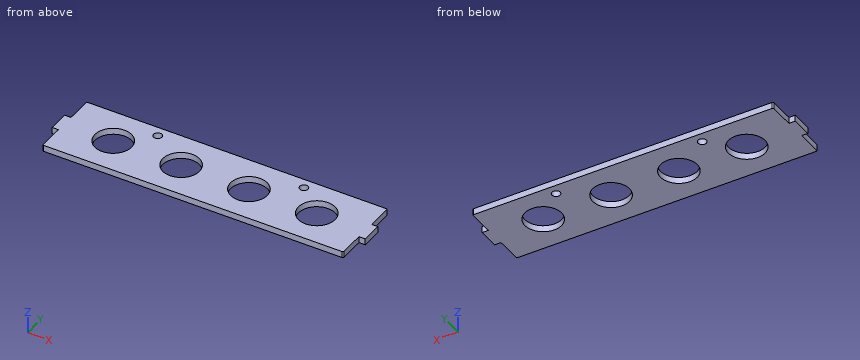
```python
from build123d import *

# Parameters (mm, degrees)
SKETCH1_W   = 300
SKETCH1_H   = 70
FRONT_DEPTH = 6
SKETCH2_W   = 6
SKETCH2_H   = 25
SKETCH2_R   = 4
MOUNT_DEPTH = 309.116860947
FILLET_2_R  = 1
SKETCH3_R   = 17.5
LITE_DEPTH  = 309.116860947


with BuildPart() as part:
    # Sketch1 → front (new body)
    with BuildSketch(Plane.XY):
        with Locations((150, 35)):
            Rectangle(SKETCH1_W, SKETCH1_H)
    extrude(amount=-FRONT_DEPTH)

    # Sketch2 → mount (cut, through all)
    with BuildSketch(Plane.XY):
        with Locations((3, 57.5)):
            Rectangle(SKETCH2_W, SKETCH2_H)
        with Locations((3, 12.5)):
            Rectangle(SKETCH2_W, SKETCH2_H)
        with Locations((297, 57.5)):
            Rectangle(SKETCH2_W, SKETCH2_H)
        with Locations((297, 12.5)):
            Rectangle(SKETCH2_W, SKETCH2_H)
        with Locations((80, 60)):
            Circle(SKETCH2_R)
        with Locations((220, 60)):
            Circle(SKETCH2_R)
    extrude(amount=-MOUNT_DEPTH, mode=Mode.SUBTRACT)

    # fillet 2
    fillet_2_edges = [part.edges().sort_by_distance(p)[0] for p in [
        (6, 70, -3),
        (6, 0, -3),
        (294, 70, -3),
        (294, 0, -3),
    ]]
    fillet(fillet_2_edges, radius=FILLET_2_R)

    # Sketch3 → lite (cut, through all)
    with BuildSketch(Plane.XY):
        with Locations((52.5, 35)):
            Circle(SKETCH3_R)
        with Locations((117.5, 35)):
            Circle(SKETCH3_R)
        with Locations((182.5, 35)):
            Circle(SKETCH3_R)
        with Locations((247.5, 35)):
            Circle(SKETCH3_R)
    extrude(amount=-LITE_DEPTH, mode=Mode.SUBTRACT)


solid = part.part
```
Model file for the job. Use its own axes, mm. Give positions to 0.01 mm unless a question says otherwise; leave off trailing zeros. Write each loop counter-clockwise with the first axis right and the second up, starting at its lowest first coordinate (ties: lowest second). Pieces come first, ordered by that corner, then holes. Notation, with made-up numbers: M 73.25,70 L 115.25,70 A12 ccw 115.25,78 Z; hole C 78,60.25 d1. An arc over 180 degrees is marked long. Use a Markdown table: item, result.
1) Cut at C-C (y = 60). List the corners of the cut face in (x, z), and give its area (3 significant figures).
Responses:
| item | result |
|---|---|
| outline | M 6,-6 L 76,-6 L 76,0 L 6,0 Z; M 84,-6 L 216,-6 L 216,0 L 84,0 Z; M 224,-6 L 294,-6 L 294,0 L 224,0 Z |
| area | 1,630 mm2 |
2) Cut at B-B (y = 35). List the corners of the cut face in (x, z), and give its area (3 significant figures).
Responses:
| item | result |
|---|---|
| outline | M 0,-6 L 35,-6 L 35,0 L 0,0 Z; M 70,-6 L 100,-6 L 100,0 L 70,0 Z; M 135,-6 L 165,-6 L 165,0 L 135,0 Z; M 200,-6 L 230,-6 L 230,0 L 200,0 Z; M 265,-6 L 300,-6 L 300,0 L 265,0 Z |
| area | 960 mm2 |
3) Pin check, flat tips, straight feed: pin 1 (1.8 mm diameter, centred on y = 57.5, z = -1.5, fed in from +X); pin 2 (3 mm diameter, centred on y = 8.5, z = -1.5, fed in from -X); pin 3 (3 mm diameter, centred on x = 2, z = -3.5, fed in from +Y). Stop position of each tip, or through.
Responses:
| item | result |
|---|---|
| pin 1 | stops at x = 294 |
| pin 2 | stops at x = 6 |
| pin 3 | stops at y = 45 |
4) Cut at A-A (x = 80). List the corners of the cut face in (y, z), and give its area (3 significant figures).
Responses:
| item | result |
|---|---|
| outline | M 0,-6 L 56,-6 L 56,0 L 0,0 Z; M 64,-6 L 70,-6 L 70,0 L 64,0 Z |
| area | 372 mm2 |
5) Drill centre lines: line 1 (Y direction, x = 182.5, z = -3.5); line 2 (X direction, y = 49.5, z = -3.05); line 3 (X direction, y = 24, z = -0.55). Where is each one in solid material? Low to high. Write a range as from..to.
Responses:
| item | result |
|---|---|
| line 1 | y = 0..17.5, 52.5..70 |
| line 2 | x = 6..42.7, 62.3..107.7, 127.3..172.7, 192.3..237.7, 257.3..294 |
| line 3 | x = 6..38.89, 66.11..103.89, 131.11..168.89, 196.11..233.89, 261.11..294 |
6) Cut at D-D (z = -3.5). List the corners of the cut face in (x, y), and give its area (3 significant figures).
Responses:
| item | result |
|---|---|
| outline | M 0,25 L 6,25 L 6,1 A1 ccw 7,0 L 293,0 A1 ccw 294,1 L 294,25 L 300,25 L 300,45 L 294,45 L 294,69 A1 ccw 293,70 L 7,70 A1 ccw 6,69 L 6,45 L 0,45 Z; hole C 52.5,35 d35; hole C 80,60 d8; hole C 117.5,35 d35; hole C 182.5,35 d35; hole C 220,60 d8; hole C 247.5,35 d35 |
| area | 16,500 mm2 |
